from build123d import *

# Parameters (mm, degrees)
F0_W     = 120
F0_H     = 35
F0_R     = 10
F1_DEPTH = 5
F2_R     = 5


with BuildPart() as f1:
    # F0 (on Top) → F1 (new body)
    with BuildSketch(Plane.XY):
        Rectangle(F0_W, F0_H)
        with Locations((-34.394763, 0)):
            Circle(F0_R, mode=Mode.SUBTRACT)
    extrude(amount=F1_DEPTH)

    # F2
    f2_edges = [f1.edges().sort_by_distance(p)[0] for p in [
        (-60, -17.5, 2.5),
        (60, 17.5, 2.5),
        (60, -17.5, 2.5),
        (-60, 17.5, 2.5),
    ]]
    fillet(f2_edges, radius=F2_R)


solid = f1.part
Model file for the job. Use its own axes, mm. Round coordinates to 2 decimals unless told otherwise and drop trailing zeros. Order: outer loops, then holes, each group sorted by start corner. A loop starts at its lowest first (then second) coordinate and runs counter-clockwise, first axis right, second up.
(1) Pull direction X, two halves, no side cores. Call faces 1 (the face through (-58.57, 16, 2.54)), 2 (the face through (-1, 0, 5)), 3 (the face through (-24.857, 3.004, 2.465)): released by +X, released by -X, zero draft, split by the parting line, or undercut.
(2) Band-saw the part on B-B (z = 3.3). List the corners of the cut face in (x, y).
(3) Band-saw the part on A-A (y = 0). List the corners of the cut face in (x, z), then the cut area to 3 significant figures.
(4) Band-saw the part on C-C (y = -8). List the corners of the cut face in (x, z).
(5) Drill centre lines: line 1 (X direction, y = -1.5, z = 4.1); line 2 (Y direction, x = -36, z = 2.6); line 3 (X direction, y = 4.5, z = 4.65). Where is each one in solid material? Low to high.
Verdict:
1. face 1: released by -X
1. face 2: zero draft
1. face 3: undercut
2. outline: (-60, -12.5) arc R5 ccw to (-55, -17.5) - (55, -17.5) arc R5 ccw to (60, -12.5) - (60, 12.5) arc R5 ccw to (55, 17.5) - (-55, 17.5) arc R5 ccw to (-60, 12.5) - close; hole circle Ø20 at (-34.39, 0)
3. outline: (-60, 0) - (-44.39, 0) - (-44.39, 5) - (-60, 5) - close; (-24.39, 0) - (60, 0) - (60, 5) - (-24.39, 5) - close
3. area: 500 mm2
4. outline: (-60, 0) - (-40.39, 0) - (-40.39, 5) - (-60, 5) - close; (-28.39, 0) - (60, 0) - (60, 5) - (-28.39, 5) - close
5. line 1: x = -60 to -44.28, -24.51 to 60
5. line 2: y = -17.5 to -9.87, 9.87 to 17.5
5. line 3: x = -60 to -43.33, -25.46 to 60
